Can you work these out from the drawing? Everything is in mm from the part's minimum corner. A direction names the side the tool comes from. Round coordinates to 2 decimals unless told otherwise and drop trailing zeros. Order: outer loops, then holes, each group sorted by start corner. A loop starts at its lowest first (then second) coordinate and runs counter-clockwise, first axis right, second up. Notation, with made-up numbers: (60.25, 61.25) - (75.25, 61.25) arc R18 ccw to (75.25, 80.25) - close; hole circle Ø4 at (-29.75, 39.25). An arc over 180 degrees is marked (long way). Answer as a JSON object with one key per item and string values.
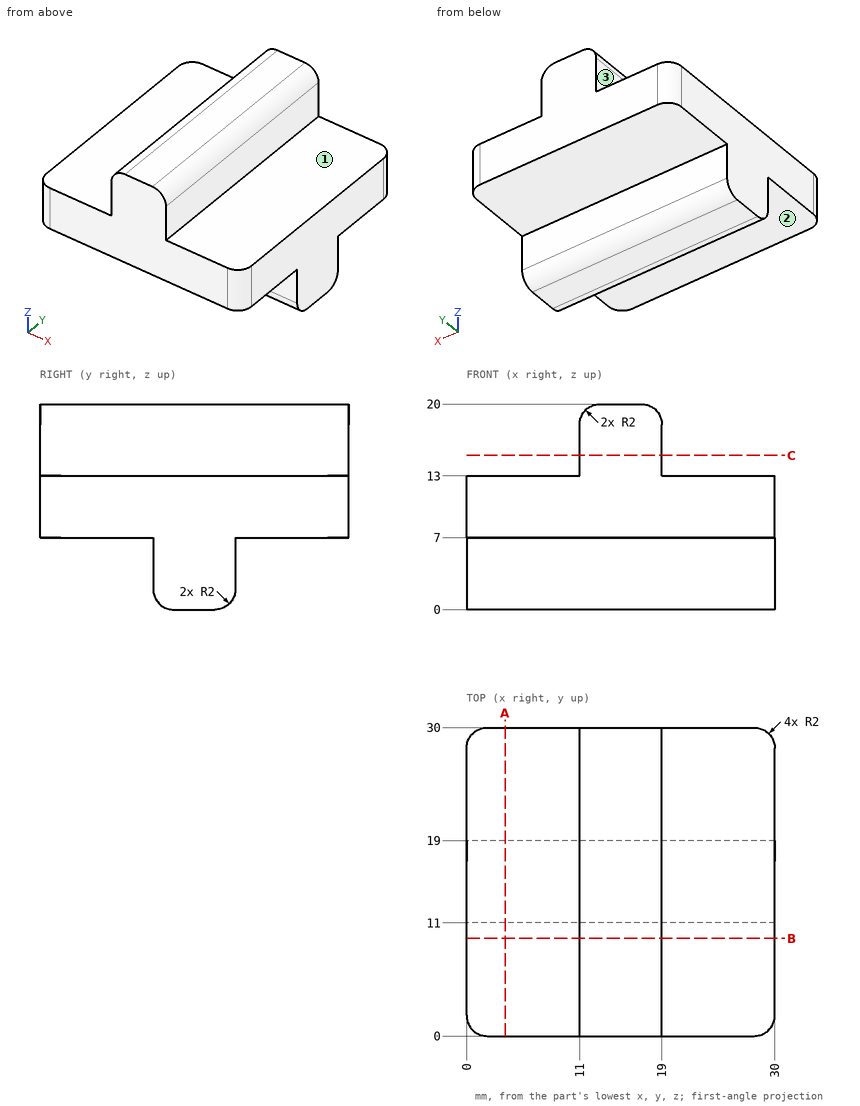
1. For P1, Ø9, axis at x = 17.5, y = 22.5, coming from the -Z side; P2, Ø5.5, axis at x = 5, y = 19, coming from the +Z side; P3, Ø3, axis at x = 21, z = 4.5, coming from the -Y side, each with a flat end and sliding along its axis, tell me the tip position at first contact or that it passes through.
Responses:
{"P1": "z = 0.27", "P2": "z = 13", "P3": "y = 11"}
2. For the marked faces 1, 2 and 3, which set-ups out of +Z, -Z, +X, -X, +Y, -Y let a thin tool reach every point of the face, with its end or its side?
Responses:
{"face 1": "+Z, +X, +Y, -Y", "face 2": "-Z, +X, -X, -Y", "face 3": "+Z, -X, +Y, -Y"}
3. Imagine slicing it at B-B (y = 9.5). List the corners of the cut face in (x, z) for me.
Responses:
{"outline": "(0, 7) - (30, 7) - (30, 13) - (19, 13) - (19, 18) arc R2 ccw to (17, 20) - (13, 20) arc R2 ccw to (11, 18) - (11, 13) - (0, 13) - close"}
4. Imagine slicing it at C-C (z = 15). List the corners of the cut face in (x, y) for me, plus the area to 3 significant figures.
Responses:
{"outline": "(11, 0) - (19, 0) - (19, 30) - (11, 30) - close", "area": "240 mm2"}
5. Imagine slicing it at A-A (x = 3.75). List the corners of the cut face in (y, z) for me, plus the area to 3 significant figures.
Responses:
{"outline": "(0, 7) - (11, 7) - (11, 2) arc R2 ccw to (13, 0) - (17, 0) arc R2 ccw to (19, 2) - (19, 7) - (30, 7) - (30, 13) - (0, 13) - close", "area": "234 mm2"}
6. If I drill on L1, parallel to X at y = 13, z = 13.25; L2, parallel to Z at x = 21.25, y = 16.25; L3, parallel to Z at x = 16.25, y = 3.5, over which ranges is the centre line in solid material (lowest first)? Write a range as [from, to].
Responses:
{"L1": "[11, 19]", "L2": "[0, 13]", "L3": "[7, 20]"}
